The figure shows three views and two pictorial views of one solid part (mm, origin at its lowest corner). Answer the questions. A direction names the side the tool comes from. Coordinates: 2 decimals unless noted, no trailing zeros. Write each loop counter-clockwise with the first axis right and the second up, starting at its lowest first coordinate (ties: lowest second). Pieces come first, ordered by that corner, then holes.
Item 1: Straight lines are drawn through the part: probe 1 along Y at (x, z) = (10, 8.5); probe 2 along Z at (x, y) = (20, 14.75); probe 3 along X at (y, z) = (16.75, 35.5). For each, find the intervals that lie inside material, in ascending order.
Item 2: Section C-C (x = 23) is taken. Give the vertices of the cut face in (y, z), then the cut area to 3 significant figures.
Item 3: Section D-D (z = 6.5) is taken. Give the vertices of the cut face in (x, y).
Item 4: A tool of negligible diameter and unlimited length cuts with its end or side. For the marked faces 1, 2 and 3, from which of +Z, -Z, +X, -X, +Y, -Y can it reach the whole face along a straight path? Write none if from no direction.
Item 5: Section B-B (z = 30) is taken. Give the vertices of the cut face in (x, y).
Item 6: Each of these flat-tipped pins is pushed along its axis until it touches: P1, Ø2, axis at y = 7.5, z = 30.5, coming from the -X side; P2, Ø4, axis at x = 27, y = 6, coming from the -Z side; P3, Ø6, axis at y = 15, z = 21.5, coming from the -X side; P4, Ø3, axis at x = 34.5, y = 8, coming from the +Z side. Where does it stop, or does it pass through?
Item 7: Section A-A (y = 16.75) is taken. Give the vertices of the cut face in (x, z), then the cut area to 3 significant figures.
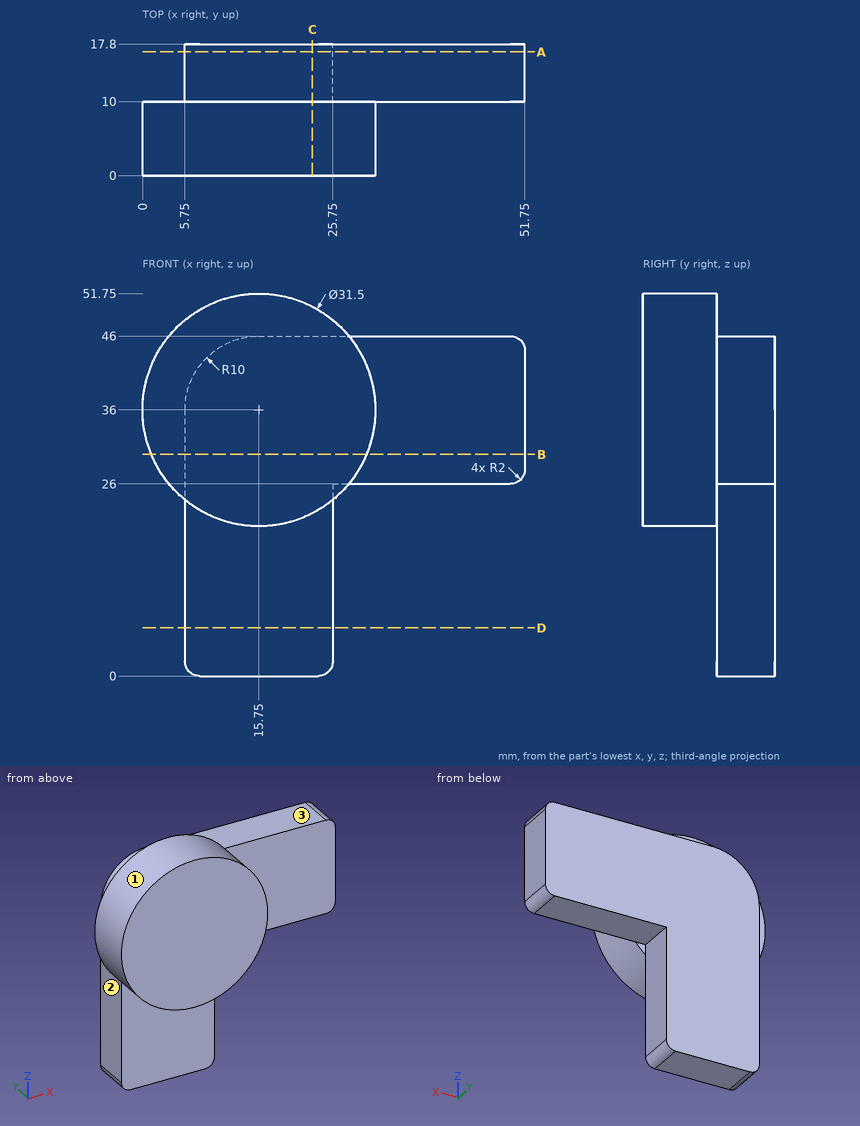
Established:
1. probe 1: y = 10 to 17.8
1. probe 2: z = 0 to 46
1. probe 3: x = 5.75 to 51.75
2. outline: (0, 22.02) - (10, 22.02) - (10, 0) - (17.8, 0) - (17.8, 46) - (10, 46) - (10, 49.98) - (0, 49.98) - close
2. area: 638 mm2
3. outline: (5.75, 10) - (25.75, 10) - (25.75, 17.8) - (5.75, 17.8) - close
4. face 1: -Y
4. face 2: +Z, -Z, -X, +Y
4. face 3: +Z, +X, -X, +Y
5. outline: (1.19, 0) - (30.31, 0) - (30.31, 10) - (51.75, 10) - (51.75, 17.8) - (5.75, 17.8) - (5.75, 10) - (1.19, 10) - close
6. P1: stops at x = 0.66
6. P2: stops at z = 23.25
6. P3: stops at x = 5.75
6. P4: passes through
7. outline: (5.75, 2) arc R2 ccw to (7.75, 0) - (23.75, 0) arc R2 ccw to (25.75, 2) - (25.75, 26) - (49.75, 26) arc R2 ccw to (51.75, 28) - (51.75, 44) arc R2 ccw to (49.75, 46) - (15.75, 46) arc R10 ccw to (5.75, 36) - close
7. area: 1,420 mm2
